Source: CAD feature listing. Evaluate the final solid. Frame: model axes, mm. Face numbers are marked on the shaded views. A direction names the side the tool comes from. Round coordinates to 2 decimals unless told otherwise and drop trailing zeros. Write each loop counter-clockwise with the first axis right and the second up, starting at its lowest first coordinate (ties: lowest second). Pieces come first, ordered by that corner, then holes.
from build123d import *

# Parameters (mm, degrees)
F0_R     = 11.15
F1_DEPTH = 7


with BuildPart() as f1:
    # F0 (on Top) → F1 (new body)
    with BuildSketch(Plane.XY):
        with BuildLine():
            ThreePointArc((11.388234, -6.575), (12.701925, -3.403471), (13.15, 0))
            ThreePointArc((13.15, 0), (12.882943, 2.636715), (12.092621, 5.166335))
            ThreePointArc((12.092621, 5.166335), (10.665576, 7.692073), (8.719458, 9.843453))
            ThreePointArc((8.719458, 9.843453), (4.662676, 12.295607), (0, 13.15))
            ThreePointArc((0, 13.15), (-5.881222, 11.761536), (-10.520488, 7.88935))
            ThreePointArc((-10.520488, 7.88935), (-11.994319, 5.390623), (-12.884409, 2.629546))
            ThreePointArc((-12.884409, 2.629546), (-12.979646, -2.109807), (-11.388234, -6.575))
            ThreePointArc((-11.388234, -6.575), (-7.245177, -10.974056), (-1.572133, -13.055684))
            ThreePointArc((-1.572133, -13.055684), (1.328743, -13.082696), (4.164951, -12.472998))
            ThreePointArc((4.164951, -12.472998), (8.31697, -10.1858), (11.388234, -6.575))
        make_face()
        Circle(F0_R, mode=Mode.SUBTRACT)
        with BuildLine():
            ThreePointArc((12.092621, 5.166335), (12.882943, 2.636715), (13.15, 0))
            ThreePointArc((13.15, 0), (12.701925, -3.403471), (11.388234, -6.575))
            ThreePointArc((11.388234, -6.575), (14.871744, -2.641059), (19.617412, -0.385093))
            ThreePointArc((19.617412, -0.385093), (16.82857, 3.710244), (12.092621, 5.166335))
        make_face()
        with BuildLine():
            ThreePointArc((9.936386, -15.988096), (9.780145, -11.145485), (11.388234, -6.575))
            ThreePointArc((11.388234, -6.575), (8.31697, -10.1858), (4.164951, -12.472998))
            ThreePointArc((4.164951, -12.472998), (7.488877, -13.511052), (9.936386, -15.988096))
        make_face()
        with BuildLine():
            ThreePointArc((19.617412, -0.385093), (14.871744, -2.641059), (11.388234, -6.575))
            ThreePointArc((11.388234, -6.575), (9.780145, -11.145485), (9.936386, -15.988096))
            ThreePointArc((9.936386, -15.988096), (24.203952, -26.222291), (35.926468, -13.15))
            ThreePointArc((35.926468, -13.15), (30.881433, -2.794709), (19.617412, -0.385093))
        make_face()
        with Locations((22.776468, -13.15)):
            Circle(F0_R, mode=Mode.SUBTRACT)
        with BuildLine():
            ThreePointArc((0, 13.15), (4.662676, 12.295607), (8.719458, 9.843453))
            ThreePointArc((8.719458, 9.843453), (7.956476, 13.241084), (8.877904, 16.59921))
            ThreePointArc((8.877904, 16.59921), (4.762201, 14.042596), (0, 13.15))
        make_face()
        with BuildLine():
            ThreePointArc((-10.520488, 7.88935), (-5.881222, 11.761536), (0, 13.15))
            ThreePointArc((0, 13.15), (-5.148648, 14.199838), (-9.475206, 17.181723))
            ThreePointArc((-9.475206, 17.181723), (-11.627451, 12.718847), (-10.520488, 7.88935))
        make_face()
        with BuildLine():
            ThreePointArc((-9.475206, 17.181723), (-5.148648, 14.199838), (0, 13.15))
            ThreePointArc((0, 13.15), (4.762201, 14.042596), (8.877904, 16.59921))
            ThreePointArc((8.877904, 16.59921), (12.034678, 21.000091), (13.15, 26.3))
            ThreePointArc((13.15, 26.3), (-4.915463, 38.496751), (-9.475206, 17.181723))
        make_face()
        with Locations((0, 26.3)):
            Circle(F0_R, mode=Mode.SUBTRACT)
        with BuildLine():
            ThreePointArc((-10.142206, -16.79663), (-5.20112, -16.429091), (-1.572133, -13.055684))
            ThreePointArc((-1.572133, -13.055684), (-7.245177, -10.974056), (-11.388234, -6.575))
            ThreePointArc((-11.388234, -6.575), (-10.074543, -9.74653), (-9.626468, -13.15))
            ThreePointArc((-9.626468, -13.15), (-9.756041, -14.99146), (-10.142206, -16.79663))
        make_face()
        with BuildLine():
            ThreePointArc((-18.81429, -0.611115), (-14.542346, -2.897111), (-11.388234, -6.575))
            ThreePointArc((-11.388234, -6.575), (-12.979646, -2.109807), (-12.884409, 2.629546))
            ThreePointArc((-12.884409, 2.629546), (-15.445353, 0.269968), (-18.81429, -0.611115))
        make_face()
        with BuildLine():
            ThreePointArc((-9.626468, -13.15), (-10.074543, -9.74653), (-11.388234, -6.575))
            ThreePointArc((-11.388234, -6.575), (-14.542346, -2.897111), (-18.81429, -0.611115))
            ThreePointArc((-18.81429, -0.611115), (-34.367551, -19.360419), (-10.142206, -16.79663))
            ThreePointArc((-10.142206, -16.79663), (-9.756041, -14.99146), (-9.626468, -13.15))
        make_face()
        with Locations((-22.776468, -13.15)):
            Circle(F0_R, mode=Mode.SUBTRACT)
    extrude(amount=F1_DEPTH)


solid = f1.part
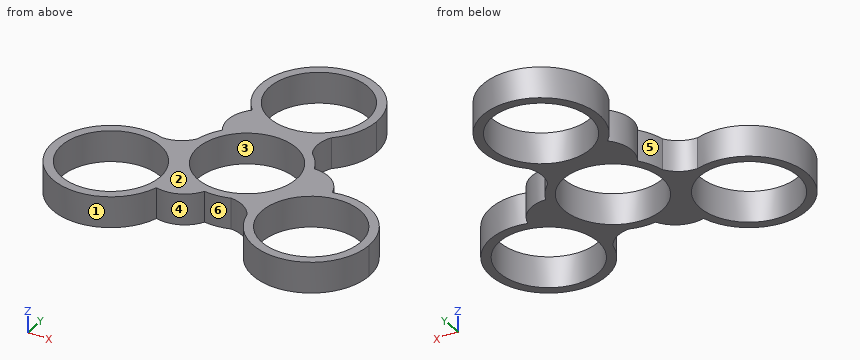
1) Material intervals for line 1 (X direction, y = -8.5, z = 5.75); line 2 (Y direction, x = -6, z = 4); line 3 (Y direction, x = 6, z = 1.75), sorted ascending.
Taken from the geometry:
line 1: x = -35.08 to -32.91, -12.64 to -7.22, 7.22 to 12.64, 32.91 to 35.08
line 2: y = -16.72 to -9.4, 9.4 to 16.9, 35.7 to 38
line 3: y = -12.82 to -9.4, 9.4 to 16.9, 35.7 to 38
2) Reachability of the marked faces 5 and 6 from +Z, -Z, +X, -X, +Y, -Y: full face, straight path, thin tool, end or side. Return the list, or none.
Taken from the geometry:
face 5: +Z, -Z, -X
face 6: +Z, -Z, -Y
3) Section query C-C on z = 1.25. Return the cut outline in (x, y).
Taken from the geometry:
outline: (-18.81, -0.61) arc R13.15 ccw (long way) to (-10.14, -16.8) arc R7.49 ccw to (-1.57, -13.06) arc R13.15 ccw to (4.16, -12.47) arc R7.2 cw to (9.94, -15.99) arc R13.15 ccw to (35.93, -13.15) arc R13.15 ccw to (19.62, -0.39) arc R7.49 ccw to (12.09, 5.17) arc R13.15 ccw to (8.72, 9.84) arc R7.2 cw to (8.88, 16.6) arc R13.15 ccw to (13.15, 26.3) arc R13.15 ccw (long way) to (-9.48, 17.18) arc R7.49 ccw to (-10.52, 7.89) arc R13.15 ccw to (-12.88, 2.63) arc R7.2 cw to start; hole circle Ø22.3 at (-22.78, -13.15); hole circle Ø22.3 at (0, 0); hole circle Ø22.3 at (0, 26.3); hole circle Ø22.3 at (22.78, -13.15)
4) Section query D-D on y = 31. Return the cut outline in (x, z), then the cut area to 3 significant figures.
Taken from the geometry:
outline: (-12.28, 0) - (-10.11, 0) - (-10.11, 7) - (-12.28, 7) - close; (10.11, 0) - (12.28, 0) - (12.28, 7) - (10.11, 7) - close
area: 30.4 mm2
5) Section query B-B on x = -29. Return the cut outline in (y, z).
Taken from the geometry:
outline: (-24.73, 0) - (-22.4, 0) - (-22.4, 7) - (-24.73, 7) - close; (-3.9, 0) - (-1.57, 0) - (-1.57, 7) - (-3.9, 7) - close
6) Section query A-A on x = 0. Return the cut outline in (y, z).
Taken from the geometry:
outline: (-13.15, 0) - (-11.15, 0) - (-11.15, 7) - (-13.15, 7) - close; (11.15, 0) - (15.15, 0) - (15.15, 7) - (11.15, 7) - close; (37.45, 0) - (39.45, 0) - (39.45, 7) - (37.45, 7) - close
7) Contact query for flat-ended pins moving along their axis: P1, Ø2, axis at x = 11, z = 6, coming from the +Y side; P2, Ø1, axis at x = -11, y = -13, coming from the -Z side; P3, Ø4, axis at y = 15.5, z = 3, coming from the +X side; P4, Ø1, axis at x = -17.5, z = 2, coming from the +Y side. Output: stop coordinate, or through.
Taken from the geometry:
P1: stops at y = 34.84
P2: stops at z = 0
P3: stops at x = 9.77
P4: stops at y = -0.36
8) Pull-direction query (Y, two-part tool) for the marked faces 1, 2, 3 and 4; classes: released by +Y, released by -Y, zero draft, split by the parting line, or undercut.
Taken from the geometry:
face 1: split by the parting line
face 2: zero draft
face 3: undercut
face 4: released by -Y
